The listing builds one solid part. Answer for the finished solid, in the listing's coordinates (mm). Face numbers are marked on the shaded views. A direction names the side the tool comes from. Coordinates: 2 decimals unless noted, no trailing zeros. Write each loop counter-clockwise with the first axis right and the second up, starting at its lowest first coordinate (ties: lowest second). Pieces come first, ordered by that corner, then holes.
from build123d import *

# Parameters (mm, degrees)
SKETCH1_R           = 1.8
BOSS_EXTRUDE1_DEPTH = 3
SKETCH2_R           = 1.8
CUT_EXTRUDE1_DEPTH  = 17.643504739
SKETCH3_W           = 25
SKETCH3_H           = 7
BOSS_EXTRUDE2_DEPTH = 3
SKETCH4_W           = 5
SKETCH4_H           = 7
BOSS_EXTRUDE3_DEPTH = 40
BOSS_EXTRUDE4_DEPTH = 7
SKETCH12_W          = 5
SKETCH12_H          = 7
BOSS_EXTRUDE5_DEPTH = 2
FILLET1_R           = 10
FILLET2_R           = 5
SKETCH13_W          = 18.381081226
SKETCH13_H          = 3.15
CUT_EXTRUDE2_DEPTH  = 12
SKETCH14_W          = 6.085668667
SKETCH14_H          = 3.15
CUT_EXTRUDE3_DEPTH  = 11


with BuildPart() as part:
    # Sketch1 → Boss-Extrude1 (new body)
    with BuildSketch(Plane(origin=(0, 0, 0), x_dir=(1, 0, 0), z_dir=(0, 1, 0))):
        with BuildLine():
            Line((-9.425, -11.725), (9.425, -11.725))
            ThreePointArc((9.425, -11.725), (10.839213562, -11.139213562), (11.425, -9.725))
            Line((11.425, -9.725), (11.425, 9.725))
            ThreePointArc((11.425, 9.725), (10.839213562, 11.139213562), (9.425, 11.725))
            Line((9.425, 11.725), (-9.425, 11.725))
            ThreePointArc((-9.425, 11.725), (-10.839213562, 11.139213562), (-11.425, 9.725))
            Line((-11.425, 9.725), (-11.425, -9.725))
            ThreePointArc((-11.425, -9.725), (-10.839213562, -11.139213562), (-9.425, -11.725))
        make_face()
        with Locations(Location((-7.925, 8.225, 0), (0, 0, 270))):
            Circle(SKETCH1_R, mode=Mode.SUBTRACT)
    extrude(amount=BOSS_EXTRUDE1_DEPTH)

    # Sketch2 → Cut-Extrude1 (cut, through all)
    with BuildSketch(Plane(origin=(0, 3, 0), x_dir=(1, 0, 0), z_dir=(0, 1, 0))):
        with Locations(Location((7.925, 8.225, 0), (0, 0, 270))):
            Circle(SKETCH2_R)
        with Locations(Location((-7.925, -8.225, 0), (0, 0, 270))):
            Circle(SKETCH2_R)
        with Locations(Location((7.925, -8.225, 0), (0, 0, 270))):
            Circle(SKETCH2_R)
    extrude(amount=-CUT_EXTRUDE1_DEPTH, mode=Mode.SUBTRACT)

    # Sketch3 → Boss-Extrude2 (add)
    with BuildSketch(Plane(origin=(0, 3, 0), x_dir=(1, 0, 0), z_dir=(0, 1, 0))):
        with Locations((12.5, 0)):
            Rectangle(SKETCH3_W, SKETCH3_H)
    extrude(amount=-BOSS_EXTRUDE2_DEPTH)

    # Sketch4 → Boss-Extrude3 (add)
    with BuildSketch(Plane.XZ):
        with Locations((22.5, 0)):
            Rectangle(SKETCH4_W, SKETCH4_H)
    extrude(amount=BOSS_EXTRUDE3_DEPTH)

    # Sketch7 → Boss-Extrude4 (add)
    with BuildSketch(Plane.XY.offset(3.5)):
        Polygon((25, 3), (35.779116369, -40.119915044), (25, -40), align=None)
    extrude(amount=-BOSS_EXTRUDE4_DEPTH)

    # Sketch12 → Boss-Extrude5 (add)
    with BuildSketch(Plane(origin=(0, 0, 0), x_dir=(1, 0, 0), z_dir=(0, 1, 0))):
        with Locations((22.5, 0)):
            Rectangle(SKETCH12_W, SKETCH12_H)
    extrude(amount=BOSS_EXTRUDE5_DEPTH)

    # Fillet1
    fillet1_edges = [part.edges().sort_by_distance(p)[0] for p in [
        (20, 0, 0),
    ]]
    fillet(fillet1_edges, radius=FILLET1_R)

    # Fillet2
    fillet2_edges = [part.edges().sort_by_distance(p)[0] for p in [
        (25, 3, 0),
    ]]
    fillet(fillet2_edges, radius=FILLET2_R)

    # Sketch13 → Cut-Extrude2 (cut)
    with BuildSketch(Plane(origin=(-0.441841569, -39.71696571, 0), x_dir=(-0.9999381256405767, 0.011124068069294642, 0), z_dir=(-0.011124068069294644, -0.9999381256405768, 0))):
        with Locations((-28.924615029, 0.005980727)):
            Rectangle(SKETCH13_W, SKETCH13_H)
    extrude(amount=-CUT_EXTRUDE2_DEPTH, mode=Mode.SUBTRACT)

    # Sketch14 → Cut-Extrude3 (cut)
    with BuildSketch(Plane.XZ.offset(40)):
        with Locations((22.485556971, 0)):
            Rectangle(SKETCH14_W, SKETCH14_H)
    extrude(amount=-CUT_EXTRUDE3_DEPTH, mode=Mode.SUBTRACT)


solid = part.part
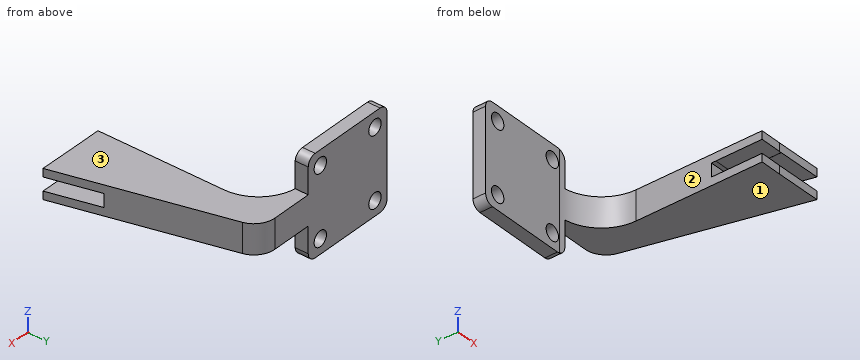
1. Section C-C on z = -2.25 is taken. Give the vertices of the cut face in (x, y) (3 decimals), then the cut area to 3 significant figures.
Results found:
outline: (-11.425, 0) - (10, 0) arc R10 cw to (20, -10) - (20, -40) - (25, -40) - (35.779, -40.12) - (25.947, -0.787) arc R5 ccw to (21.096, 3) - (-11.425, 3) - close
area: 560 mm2
2. Section B-B on y = -32.5 is taken. Give the vertices of the cut face in (x, z) (3 decimals), then the cut area to 3 significant figures.
Results found:
outline: (20, -3.5) - (33.874, -3.5) - (33.874, -1.581) - (20, -1.581) - close; (20, 1.575) - (25.528, 1.575) - (25.528, 1.569) - (33.874, 1.569) - (33.874, 3.5) - (20, 3.5) - close
area: 53.4 mm2
3. Find the intervals of material crossed by L1, parallel to Y at x = 3.5, z = -10.5; L2, parallel to Z at x = 22, y = -14; L3, parallel to Y at x = 12, z = -1, in increasing order.
Results found:
L1: y = 0 to 3
L2: z = -3.5 to 3.5
L3: y = -0.2 to 3
4. Flat-ended cylindrical pins translate along their axes: P1, Ø1.5, axis at x = 22, z = -2.5, coming from the -Y side; P2, Ø3.5, axis at y = -21.5, z = 0, coming from the -X side; P3, Ø7.5, axis at x = 28, y = -26, coming from the +Z side. Find the tip coordinate at first contact, or state that the pin passes through.
Results found:
P1: stops at y = -40
P2: stops at x = 20
P3: stops at z = 3.5
5. Section A-A on z = 9 is taken. Give the vertices of the cut face in (x, y) (3 decimals).
Results found:
outline: (-11.425, 0) - (-9.55, 0) - (-9.55, 3) - (-11.425, 3) - close; (-6.3, 0) - (6.3, 0) - (6.3, 3) - (-6.3, 3) - close; (9.55, 0) - (10, 0) arc R10 cw to (11.425, -0.102) - (11.425, 3) - (9.55, 3) - close
6. Section D-D on x = 22 is taken. Give the vertices of the cut face in (y, z) (3 decimals).
Results found:
outline: (-40, -3.5) - (2.918, -3.5) - (2.918, 3.5) - (-40, 3.5) - (-40, 1.575) - (-29, 1.575) - (-29, 1.569) - (-27.966, 1.569) - (-27.966, -1.581) - (-39.967, -1.581) - (-39.967, -1.575) - (-40, -1.575) - close
7. A tool of negligible diameter and unlimited length cuts with its end or side. For the marked faces 1, 2 and 3, from which of +Z, -Z, +X, -X, +Y, -Y can it reach the whole face along a straight path? Write none if from no direction.
Results found:
face 1: -Z, +X, +Y, -Y
face 2: +Z, -Z, -X, -Y
face 3: +Z, +X, +Y, -Y
